```python
from build123d import *

# Parameters (mm, degrees)
SKETCH1_R                    = 12.2
BOSS_EXTRUDE1_DEPTH          = 13
M1_6_CLEARANCE_HOLE2_D       = 1.8
F_3_8_0_375_DIAMETER_HOLE1_D = 9.525
CUT_EXTRUDE1_START           = 1
SKETCH1_4_R                  = 12.2
CUT_EXTRUDE1_DEPTH           = 43.751089129
BOSS_EXTRUDE2_DEPTH          = 3.175
F_10_CLEARANCE_HOLE1_D       = 5.1054
FILLET1_R                    = 1.651
CUT_EXTRUDE2_DEPTH           = 52.305959936
CUT_EXTRUDE3_DEPTH           = 52.305959936
FILLET2_R                    = 1.905
CUT_EXTRUDE4_DEPTH           = 1.5875


with BuildPart() as part:
    # Sketch1 → Boss-Extrude1 (new body)
    # profile 1 of 2: a face of its own
    with BuildSketch(Plane.XY):
        with BuildLine():
            Line((25.4, 13.97), (-25.4, 13.97))
            ThreePointArc((-25.4, 13.97), (-39.37, 0), (-25.4, -13.97))
            Line((-25.4, -13.97), (25.4, -13.97))
            ThreePointArc((25.4, -13.97), (39.37, 0), (25.4, 13.97))
        make_face()
        with Locations((-25.4, 0)):
            Circle(SKETCH1_R, mode=Mode.SUBTRACT)
    # profile 2 of 2: a face of its own
    with BuildSketch(Plane.XY):
        with Locations((-25.4, 0)):
            Circle(SKETCH1_R)
    extrude(amount=BOSS_EXTRUDE1_DEPTH)

    # M1.6 Clearance Hole2 (through all)
    with Locations(Plane.XY.offset(13)):
        with Locations((-32.32820323, 4), (-25.4, 8), (-18.47179677, 4), (-18.47179677, -4), (-25.4, -8), (-32.32820323, -4)):
            Hole(M1_6_CLEARANCE_HOLE2_D / 2)

    # 3_8 _0.375_ Diameter Hole1 (through all)
    with Locations(Plane.XY.offset(13)):
        with Locations((25.4, 0)):
            Hole(F_3_8_0_375_DIAMETER_HOLE1_D / 2)

    # Sketch1_4 → Cut-Extrude1 (cut, through all)
    with BuildSketch(Plane.XY.offset(CUT_EXTRUDE1_START)):
        with Locations((-25.4, 0)):
            Circle(SKETCH1_4_R)
    extrude(amount=CUT_EXTRUDE1_DEPTH, mode=Mode.SUBTRACT)

    # Sketch7 → Boss-Extrude2 (add, symmetric)
    with BuildSketch(Plane(origin=(0, 0, 0), x_dir=(1, 0, 0), z_dir=(0, 1, 0))):
        Polygon((-38.1, 0), (-47.625, 0), (-47.625, -9.525), (-42.8625, -9.525), (-42.8625, -13), (-38.1, -13), align=None)
    extrude(amount=BOSS_EXTRUDE2_DEPTH, both=True)

    # 10 Clearance Hole1 (through all)
    with Locations(Plane(origin=(0, -3.175, 0), x_dir=(-1, 0, 0), z_dir=(0, -1, 0))):
        with Locations((43.314710578, -4.7625)):
            Hole(F_10_CLEARANCE_HOLE1_D / 2)

    # Fillet1
    fillet1_edges = [part.edges().sort_by_distance(p)[0] for p in [
        (-47.625, 0, 0),
        (-47.625, 0, 9.525),
        (-42.8625, 0, 9.525),
        (-42.8625, 0, 13),
    ]]
    fillet(fillet1_edges, radius=FILLET1_R)

    # Sketch9 → Cut-Extrude2 (cut, through all)
    with BuildSketch(Plane.XY.offset(13)):
        with BuildLine():
            Line((-29.095845641, 0.635), (-47.625, 0.635))
            Line((-47.625, 0.635), (-47.625, -0.635))
            Line((-47.625, -0.635), (-29.095845641, -0.635))
            ThreePointArc((-29.095845641, -0.635), (-29.15, 0), (-29.095845641, 0.635))
        make_face()
        with BuildLine():
            ThreePointArc((-29.095845641, -0.635), (-21.65, 0), (-29.095845641, 0.635))
            ThreePointArc((-29.095845641, 0.635), (-29.15, 0), (-29.095845641, -0.635))
        make_face()
    extrude(amount=-CUT_EXTRUDE2_DEPTH, mode=Mode.SUBTRACT)

    # Sketch13 → Cut-Extrude3 (cut, through all)
    with BuildSketch(Plane.XY.offset(13)):
        with BuildLine():
            Line((-16.532707572, 10.795), (16.532707572, 10.795))
            ThreePointArc((16.532707572, 10.795), (11.43, 0), (16.532707572, -10.795))
            Line((16.532707572, -10.795), (-16.532707572, -10.795))
            ThreePointArc((-16.532707572, -10.795), (-11.43, 0), (-16.532707572, 10.795))
        make_face()
    extrude(amount=-CUT_EXTRUDE3_DEPTH, mode=Mode.SUBTRACT)

    # Fillet2
    fillet2_edges = [part.edges().sort_by_distance(p)[0] for p in [
        (-16.532707572, -10.795, 6.5),
        (-16.532707572, 10.795, 6.5),
        (16.532707572, 10.795, 6.5),
        (16.532707572, -10.795, 6.5),
    ]]
    fillet(fillet2_edges, radius=FILLET2_R)

    # Sketch14 → Cut-Extrude4 (cut)
    with BuildSketch(Plane.XY.offset(13)):
        with BuildLine():
            Line((-25.4, 1.5875), (0, 1.5875))
            ThreePointArc((0, 1.5875), (1.5875, 0), (0, -1.5875))
            Line((0, -1.5875), (-25.4, -1.5875))
            ThreePointArc((-25.4, -1.5875), (-26.9875, 0), (-25.4, 1.5875))
        make_face()
    extrude(amount=-CUT_EXTRUDE4_DEPTH, mode=Mode.SUBTRACT)


solid = part.part
```
Here's how the part is built. I have some questions about the finished solid (model axes, mm). A direction names the side the tool comes from. Coordinates: 2 decimals unless noted, no trailing zeros. Loops run counter-clockwise (first coordinate to the right, second up) from the corner with the lowest first, then second, coordinate; pieces in that order, holes last. Notation, with made-up numbers: M 33,-4.5 L 71,-4.5 A17 cw 71,24.5 Z; hole C -20.75,74 d5. An arc over 180 degrees is marked long. One line per item, written item: value.
1. Imagine slicing it at C-C (y = -6). List the corners of the cut face in (x, z) for me.
Geometry says:
outline: M -38.02,0 L -12.78,0 L -12.78,13 L -14.78,13 L -14.78,1 L -36.02,1 L -36.02,13 L -38.02,13 Z; M 12.78,0 L 38.02,0 L 38.02,13 L 12.78,13 Z
2. Will these pins go through, and if not, where does the flat tip stop? pin 1 Ø4 at (y, z) = (4.5, 7.5) entering from +X; pin 2 Ø2.5 at (x, z) = (-44.5, 4) entering from -Y (3 decimals); pin 3 Ø14.5 at (x, y) = (-25.4, 0) entering from +Z.
Geometry says:
pin 1: stops at x = 39.14
pin 2: stops at y = -3.175
pin 3: stops at z = 1
3. Imagine slicing it at D-D (x = 21.5). List the corners of the cut face in (y, z) for me, and give its area (3 significant figures).
Geometry says:
outline: M -13.97,0 L -2.73,0 L -2.73,13 L -13.97,13 Z; M 2.73,0 L 13.97,0 L 13.97,13 L 2.73,13 Z
area: 292 mm2
4. Please list where these lines run through material, in increasing order: probe 1 along Y at (x, z) = (-25.4, 0.55); probe 2 along X at (y, z) = (-8, 4); probe 3 along X at (y, z) = (-8.5, 9).
Geometry says:
probe 1: y = -13.97 to -8.9, -7.1 to -3.75, 3.75 to 7.1, 8.9 to 13.97
probe 2: x = -36.85 to -34.61, -16.19 to -13.93, 13.93 to 36.85
probe 3: x = -36.49 to -34.15, -16.65 to -14.11, 14.11 to 36.49
5. Imagine slicing it at A-A (x = 1.5). List the corners of the cut face in (y, z) for me (3 decimals), and give its area (4 significant figures).
Geometry says:
outline: M -13.97,0 L -10.795,0 L -10.795,13 L -13.97,13 Z; M 10.795,0 L 13.97,0 L 13.97,13 L 10.795,13 Z
area: 82.55 mm2
6. On a 3-axis mill with a long thin cutter (end or side, diameter ignored), from which of +Z, -Z, +X, -X, +Y, -Y can I reach the whole of each face in a straight line? I mean faces 4 (the flat face through (-28, -3, 1)), 5 (the cylindrical face through (-13.943, -9.758, 6.409)), 6 (the flat face through (-43, 3.175, 8)). Say none if no direction works.
Geometry says:
face 4: +Z
face 5: +Z, -Z
face 6: +Z, -Z, -X, +Y
7. Imagine slicing it at B-B (z = 3.75). State how many separate pieces and enclosed holes the cut face has, and give its area (3 significant figures).
Geometry says:
separate pieces: 3
enclosed holes: 2
area: 964 mm2
8. Thinking about a two-plate mould opening in Y: for faces 1 (the flat face through (0, 13.97, 6)), 2 (the cylindrical face through (-11.43, -0.12, 6.59)), 3 (the cylindrical face through (-43.333, 1.923, 10.021)), which applies, +Y half, -Y half, draft (parallel to the pull), parting line (faces both ways), or undercut?
Geometry says:
face 1: +Y half
face 2: undercut
face 3: draft
